Input: part model. Units: mm. Frame: model coordinates. Round coordinates to 2 decimals unless told otherwise and drop trailing zeros. Loops run counter-clockwise (first coordinate to the right, second up) from the corner with the lowest first, then second, coordinate; pieces in that order, holes last. Notation, with made-up numbers: (14.25, 68) - (68.25, 68) arc R18 cw to (68.25, 78) - close; hole circle Ø10 at (86.25, 2.5). An arc over 180 degrees is marked (long way). Write each question's results on one line, items separated by ' | '.
from build123d import *

# Parameters (mm, degrees)
F2_R = 3.175


with BuildPart() as f3:
    # F3: sweep along a path in F0
    with BuildLine(Plane.XY) as f3_path:
        Line((127, 152.4), (127, 12.7))
        ThreePointArc((127, 12.7), (123.2802561211, 3.7197438789), (114.3, 0))
        Line((114.3, 0), (12.7, 0))
        ThreePointArc((12.7, 0), (3.7197438789, -3.7197438789), (0, -12.7))
        Line((0, -12.7), (0, -114.3))
        ThreePointArc((0, -114.3), (12.7, -127), (25.4, -114.3))
        Line((25.4, -114.3), (25.4, -38.1))
        ThreePointArc((25.4, -38.1), (29.1197438789, -29.1197438789), (38.1, -25.4))
        Line((38.1, -25.4), (127, -25.4))
    # F2 (on offset) → F3 (sweep)
    with BuildSketch(Plane.XZ.offset(-152.4)):
        with Locations((127, 0)):
            Circle(F2_R)
    sweep(path=f3_path.line)


solid = f3.part
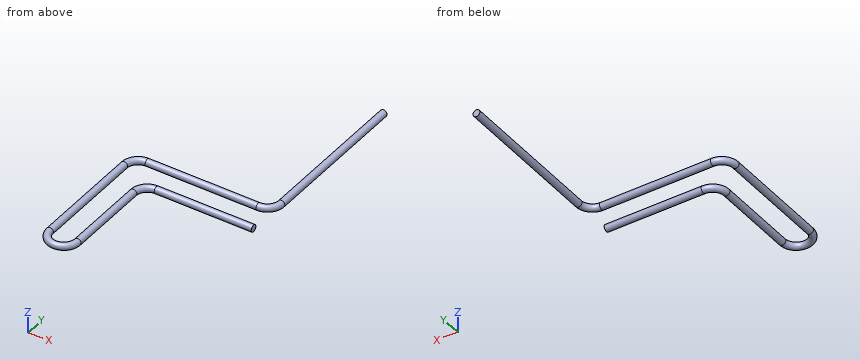
1. Contact query for flat-ended pins moving along their axis: pin 1 (12 mm diameter, centred on x = 18, y = -62, fed in from -Z); pin 2 (3 mm diameter, centred on y = 42.5, z = 0.5, fed in from +X) (3 decimals); pin 3 (3 mm diameter, centred on x = 12.5, z = 2, fed in from +Y); pin 4 (2 mm diameter, centred on y = 69, z = 2.5, fed in from +X). Output: stop coordinate, or through.
Answer:
pin 1: z = -2.85 | pin 2: x = 130.175 | pin 3: y = 3.13 | pin 4: x = 129.8
2. Line query: line 1 (Y direction, x = 98, z = 0) (3 decimals); line 2 (Y direction, x = 90, z = -2.25); line 3 (X direction, y = -39, z = -0.75). Output: solid intervals per line, ascending. Write a range as [from, to].
Answer:
line 1: [-28.575, -22.225], [-3.175, 3.175] | line 2: [-27.64, -23.16], [-2.24, 2.24] | line 3: [-3.09, 3.09], [22.31, 28.49]
3. Section query B-B, the plane x = 68. Output: boundary loops of the cut face in (y, z) (3 decimals).
Answer:
outline: circle Ø6.35 at (-25.4, 0); circle Ø6.35 at (0, 0)
4. Section query A-A, the plane z = 0. Output: boundary loops of the cut face in (x, y) (3 decimals), plus the area to 3 significant figures.
Answer:
outline: (-3.175, -114.3) arc R15.875 ccw to (28.575, -114.3) - (28.575, -38.1) arc R9.525 cw to (38.1, -28.575) - (127, -28.575) - (127, -22.225) - (38.1, -22.225) arc R15.875 ccw to (22.225, -38.1) - (22.225, -114.3) arc R9.525 cw to (3.175, -114.3) - (3.175, -12.7) arc R9.525 cw to (12.7, -3.175) - (114.3, -3.175) arc R15.875 ccw to (130.175, 12.7) - (130.175, 152.4) - (123.825, 152.4) - (123.825, 12.7) arc R9.525 cw to (114.3, 3.175) - (12.7, 3.175) arc R15.875 ccw to (-3.175, -12.7) - close | area: 3,860 mm^2
5. Section query C-C, the plane y = 68.5. Output: boundary loops of the cut face in (x, z) (3 decimals).
Answer:
outline: circle Ø6.35 at (127, 0)
